Print and shaded views of the part. All mm, measured from the part's lowest x, y and z. Round coordinates to 2 decimals unless told otherwise and drop trailing zeros. Write each loop counter-clockwise with the first axis right and the second up, starting at its lowest first coordinate (ties: lowest second). Pieces come first, ordered by that corner, then holes. Notation, with made-up numbers: M 74,80.5 L 85,80.5 A30 ccw 85,102.5 Z; hole C 55,33.5 d4. An arc over 180 degrees is marked long. Write item = value, one per line. Start each with the question number.
Q1. Band-saw the part on A-A on z = 10. Write the cut outline in (x, y), plus the area to 3 significant figures.
Q2. Band-saw the part on B-B on x = 80. Write the cut outline in (y, z).
Q3. Band-saw the part on D-D on z = 50. Write the cut outline in (x, y).
Q4. Band-saw the part on C-C on x = 40. Write the cut outline in (y, z).
Q5. Drop a flat-ended pin along its axis: P1, Ø5.5, axis at x = 20, z = 90, coming from the -Y side. Give the stop position or say it passes through.
Q6. Probe L1, parallel to X at y = 8, z = 90; L2, parallel to X at y = 12.25, z = 50; L3, parallel to Z at x = 79, y = 1.25. List the from-to ranges inside material, lowest first.
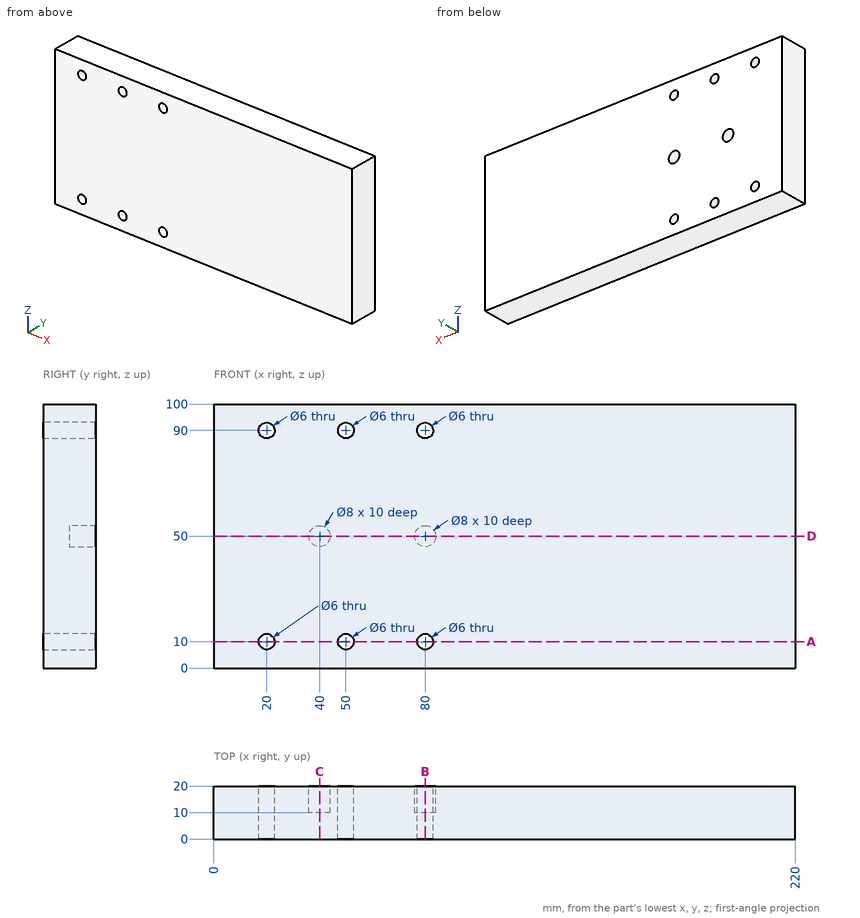
Conclusion:
q1.outline = M 0,0 L 17,0 L 17,20 L 0,20 Z; M 23,0 L 47,0 L 47,20 L 23,20 Z; M 53,0 L 77,0 L 77,20 L 53,20 Z; M 83,0 L 220,0 L 220,20 L 83,20 Z
q1.area = 4,040 mm^2
q2.outline = M 0,0 L 20,0 L 20,7 L 0,7 Z; M 0,13 L 20,13 L 20,46 L 10,46 L 10,54 L 20,54 L 20,87 L 0,87 Z; M 0,93 L 20,93 L 20,100 L 0,100 Z
q3.outline = M 0,0 L 220,0 L 220,20 L 84,20 L 84,10 L 76,10 L 76,20 L 44,20 L 44,10 L 36,10 L 36,20 L 0,20 Z
q4.outline = M 0,0 L 20,0 L 20,46 L 10,46 L 10,54 L 20,54 L 20,100 L 0,100 Z
q5.P1 = through
q6.L1 = 0 to 17, 23 to 47, 53 to 77, 83 to 220
q6.L2 = 0 to 36, 44 to 76, 84 to 220
q6.L3 = 0 to 7.17, 12.83 to 87.17, 92.83 to 100
